```python
from build123d import *

# Parameters (mm, degrees)
SKETCH1_R           = 2.54
SKETCH1_R_2         = 1.905
BOSS_EXTRUDE1_DEPTH = 3.81
SKETCH4_R           = 3.556
SKETCH4_R_2         = 1.905
BOSS_EXTRUDE4_DEPTH = 11.176


with BuildPart() as part:
    # Sketch1 → Boss-Extrude1 (new body)
    with BuildSketch(Plane(origin=(0, 0, 0), x_dir=(1, 0, 0), z_dir=(0, 1, 0))):
        with BuildLine():
            Line((-9.948186072, 14.224), (-9.948186072, -14.224))
            ThreePointArc((-9.948186072, -14.224), (-6.392186072, -17.78), (-2.836186072, -14.224))
            Line((-2.836186072, -14.224), (-2.836186072, -5.08))
            Line((-2.836186072, -5.08), (5.799813928, -5.08))
            Line((5.799813928, -5.08), (5.799813928, -14.224))
            ThreePointArc((5.799813928, -14.224), (9.355813928, -17.78), (12.911813928, -14.224))
            Line((12.911813928, -14.224), (12.911813928, 14.224))
            ThreePointArc((12.911813928, 14.224), (9.355813928, 17.78), (5.799813928, 14.224))
            Line((5.799813928, 14.224), (5.799813928, 5.08))
            Line((5.799813928, 5.08), (-2.836186072, 5.08))
            Line((-2.836186072, 5.08), (-2.836186072, 14.224))
            ThreePointArc((-2.836186072, 14.224), (-6.392186072, 17.78), (-9.948186072, 14.224))
        make_face()
        with Locations(Location((7.831813928, 0, 0), (0, 0, 90))):
            Circle(SKETCH1_R, mode=Mode.SUBTRACT)
        with Locations(Location((-4.868186072, 0, 0), (0, 0, 90))):
            Circle(SKETCH1_R, mode=Mode.SUBTRACT)
        with Locations(Location((-6.392186072, 14.224, 0), (0, 0, 90))):
            Circle(SKETCH1_R_2, mode=Mode.SUBTRACT)
        with Locations(Location((-6.392186072, -14.224, 0), (0, 0, 90))):
            Circle(SKETCH1_R_2, mode=Mode.SUBTRACT)
        with Locations(Location((9.355813928, 14.224, 0), (0, 0, 90))):
            Circle(SKETCH1_R_2, mode=Mode.SUBTRACT)
        with Locations(Location((9.355813928, -14.224, 0), (0, 0, 90))):
            Circle(SKETCH1_R_2, mode=Mode.SUBTRACT)
    extrude(amount=BOSS_EXTRUDE1_DEPTH)

    # Sketch4 → Boss-Extrude4 (add)
    # profile 1 of 4: a face of its own
    with BuildSketch(Plane(origin=(0, 3.81, 0), x_dir=(1, 0, 0), z_dir=(0, 1, 0))):
        with Locations(Location((-6.392186072, 14.224, 0), (0, 0, 180))):
            Circle(SKETCH4_R)
        with Locations(Location((-6.392186072, 14.224, 0), (0, 0, 90))):
            Circle(SKETCH4_R_2, mode=Mode.SUBTRACT)
    # profile 2 of 4: a face of its own
    with BuildSketch(Plane(origin=(0, 3.81, 0), x_dir=(1, 0, 0), z_dir=(0, 1, 0))):
        with Locations(Location((9.355813928, 14.224, 0), (0, 0, 180))):
            Circle(SKETCH4_R)
        with Locations(Location((9.355813928, 14.224, 0), (0, 0, 90))):
            Circle(SKETCH4_R_2, mode=Mode.SUBTRACT)
    # profile 3 of 4: a face of its own
    with BuildSketch(Plane(origin=(0, 3.81, 0), x_dir=(1, 0, 0), z_dir=(0, 1, 0))):
        with Locations((9.355813928, -14.224)):
            Circle(SKETCH4_R)
        with Locations(Location((9.355813928, -14.224, 0), (0, 0, 90))):
            Circle(SKETCH4_R_2, mode=Mode.SUBTRACT)
    # profile 4 of 4: a face of its own
    with BuildSketch(Plane(origin=(0, 3.81, 0), x_dir=(1, 0, 0), z_dir=(0, 1, 0))):
        with Locations((-6.392186072, -14.224)):
            Circle(SKETCH4_R)
        with Locations(Location((-6.392186072, -14.224, 0), (0, 0, 90))):
            Circle(SKETCH4_R_2, mode=Mode.SUBTRACT)
    extrude(amount=BOSS_EXTRUDE4_DEPTH)


solid = part.part
```
Build history of the part. All positions in model axes, mm. A direction names the side the tool comes from. Coordinates: 2 decimals unless noted, no trailing zeros. Order: outer loops, then holes, each group sorted by start corner. A loop starts at its lowest first (then second) coordinate and runs counter-clockwise, first axis right, second up. Notation, with made-up numbers: (2, 50) -> (17, 50) arc R23 cw to (17, 63) -> close; hole circle Ø1 at (-14.5, 68). An arc over 180 degrees is marked (long way). Answer in a Markdown table with one row per item. Add a question column.
Q1. Band-saw the part on C-C, the plane z = 0. List the corners of the cut face in (x, y), then the cut area to 3 significant figures.
Q2. Wall check: line 1 along X through (y, z) = (2.7, 0); line 2 along Z through (x, y) = (9, 12.25); line 3 along Z through (x, y) = (7.75, 8.5). Give the ranges that are in metal, low to high. Write a range as [from, to].
Q3. Band-saw the part on D-D, the plane y = 2.5. List the corners of the cut face in (x, z) (3 decimals), then the cut area to 3 significant figures.
Q4. Band-saw the part on B-B, the plane y = 12.5. List the corners of the cut face in (x, z) (3 decimals).
Q5. Mould opens along X. For faces 1 (the face through (-7.387, 1.878, 0.331)), 2 (the face through (11, 14.986, 16)), 3 (the face through (10.085, 7.388, 12.464)), 4 (the face through (-9.948, 2, 0)) say: +X half, -X half, draft (parallel to the pull), parting line (faces both ways), or undercut.
Q6. Band-saw the part on A-A, the plane z = 6.5. List the corners of the cut face in (x, y).
Q7. Which spindle directions (+Z, -Z, +X, -X, +Y, -Y) get a long thin tool onto all of the face, cutting with end or side? Do faces 5 (the face through (1, 2, 5.08)), 6 (the face through (-7.163, 7.388, 17.695)), 7 (the face through (2, 2, -5.08)). Say none if no direction does.
Q8. Drop flat-ended pins along their axis: pin 1 (6 mm diameter, centred on x = -4.87, z = 0, fed in from +Y); pin 2 (1.5 mm diameter, centred on x = 5.5, y = 12.5, fed in from -Z); pin 3 (4 mm diameter, centred on x = 3.5, y = 2.5, fed in from +Z). Give the stop position or say it passes through.
Answers follow:
| question | item | result |
|---|---|---|
| 1 | outline | (-9.95, 0) -> (-7.41, 0) -> (-7.41, 3.81) -> (-9.95, 3.81) -> close; (-2.33, 0) -> (5.29, 0) -> (5.29, 3.81) -> (-2.33, 3.81) -> close; (10.37, 0) -> (12.91, 0) -> (12.91, 3.81) -> (10.37, 3.81) -> close |
| 1 | area | 48.4 mm^2 |
| 2 | line 1 | [-9.95, -7.41], [-2.33, 5.29], [10.37, 12.91] |
| 2 | line 2 | [-17.76, -16.1], [-12.35, -10.69], [10.69, 12.35], [16.1, 17.76] |
| 2 | line 3 | [-17.4, -15.25], [-13.2, -11.05], [11.05, 13.2], [15.25, 17.4] |
| 3 | outline | (-9.948, -14.224) arc R3.556 ccw to (-2.836, -14.224) -> (-2.836, -5.08) -> (5.8, -5.08) -> (5.8, -14.224) arc R3.556 ccw to (12.912, -14.224) -> (12.912, 14.224) arc R3.556 ccw to (5.8, 14.224) -> (5.8, 5.08) -> (-2.836, 5.08) -> (-2.836, 14.224) arc R3.556 ccw to (-9.948, 14.224) -> close; hole circle Ø3.81 at (-6.392, -14.224); hole circle Ø3.81 at (-6.392, 14.224); hole circle Ø5.08 at (-4.868, 0); hole circle Ø5.08 at (7.832, 0); hole circle Ø3.81 at (9.356, -14.224); hole circle Ø3.81 at (9.356, 14.224) |
| 3 | area | 486 mm^2 |
| 4 | outline | circle Ø7.112 at (-6.392, -14.224); circle Ø7.112 at (-6.392, 14.224); circle Ø7.112 at (9.356, -14.224); circle Ø7.112 at (9.356, 14.224); hole circle Ø3.81 at (-6.392, -14.224); hole circle Ø3.81 at (-6.392, 14.224); hole circle Ø3.81 at (9.356, -14.224); hole circle Ø3.81 at (9.356, 14.224) |
| 5 | face 1 | undercut |
| 5 | face 2 | draft |
| 5 | face 3 | undercut |
| 5 | face 4 | -X half |
| 6 | outline | (-9.95, 0) -> (-2.84, 0) -> (-2.84, 3.81) -> (-9.95, 3.81) -> close; (5.8, 0) -> (12.91, 0) -> (12.91, 3.81) -> (5.8, 3.81) -> close |
| 7 | face 5 | +Z, +Y, -Y |
| 7 | face 6 | +Y |
| 7 | face 7 | -Z, +Y, -Y |
| 8 | pin 1 | y = 3.81 |
| 8 | pin 2 | z = -15.96 |
| 8 | pin 3 | z = 5.08 |
